Here's how the part is built. I have some questions about the finished solid (model axes, mm). Coordinates: 2 decimals unless noted, no trailing zeros. Use one line per item in the form item = value. Start each with the question number.
(1) Thinking about a two-plate mould opening in Z: for faces 1 (the cylindrical face through (40.926, 1.479, -84.608)), 2 (the flat face through (12, 3, -54)), 3 (the cylindrical face through (13.16, 1.48, 31.19)), 4 (the cylindrical face through (-39.44, 1.52, 36.02)), which applies, +Z half, -Z half, draft (parallel to the pull), parting line (faces both ways), or undercut?
(2) Imagine slicing it at A-A, the plane y = 0.8. State how many separate pieces and enclosed holes the cut face has, and give its area (3 significant figures).
(3) Please list where these lines run through material, in increasing order: L1, parallel to Z at x = 3, y = 1.4; L2, parallel to Z at x = 14, y = 2.3; L3, parallel to Z at x = 62, y = 0.4.
(4) Will these pins go through, and if not, where does the flat tip stop? P1, Ø4, axis at x = 12.63, z = -10.48, coming from the +Y side; P2, Ø2, axis at x = 32.63, z = 29.52, coming from the -Y side.
```python
from build123d import *

# Parameters (mm, degrees)
SKETCH1_W           = 107
SKETCH1_H           = 179.75
SKETCH1_R           = 1.75
BOSS_EXTRUDE1_DEPTH = 3
FILLET1_R           = 5


with BuildPart() as part:
    # Sketch1 → Boss-Extrude1 (new body)
    with BuildSketch(Plane(origin=(0, 0, 0), x_dir=(1, 0, 0), z_dir=(0, 1, 0))):
        with Locations((12.634153991, 52.353571429)):
            Rectangle(SKETCH1_W, SKETCH1_H)
        with Locations(Location((-32.865846009, -22.771428571, 0), (0, 0, 270))):
            Circle(SKETCH1_R, mode=Mode.SUBTRACT)
        with Locations(Location((-32.865846009, 59.728571429, 0), (0, 0, 270))):
            Circle(SKETCH1_R, mode=Mode.SUBTRACT)
        with Locations(Location((-32.865846009, -29.521428571, 0), (0, 0, 270))):
            Circle(SKETCH1_R, mode=Mode.SUBTRACT)
        with Locations(Location((-32.865846009, -16.021428571, 0), (0, 0, 270))):
            Circle(SKETCH1_R, mode=Mode.SUBTRACT)
        with Locations(Location((-32.865846009, 22.978571429, 0), (0, 0, 270))):
            Circle(SKETCH1_R, mode=Mode.SUBTRACT)
        with Locations(Location((-32.865846009, 30.478571429, 0), (0, 0, 270))):
            Circle(SKETCH1_R, mode=Mode.SUBTRACT)
        with Locations(Location((-32.865846009, 71.728571429, 0), (0, 0, 270))):
            Circle(SKETCH1_R, mode=Mode.SUBTRACT)
        with Locations(Location((-32.865846009, 84.228571429, 0), (0, 0, 270))):
            Circle(SKETCH1_R, mode=Mode.SUBTRACT)
        with Locations(Location((-32.865846009, 104.728571429, 0), (0, 0, 270))):
            Circle(SKETCH1_R, mode=Mode.SUBTRACT)
        with Locations(Location((12.634153991, 84.228571429, 0), (0, 0, 270))):
            Circle(SKETCH1_R, mode=Mode.SUBTRACT)
        with Locations(Location((2.634153991, 84.228571429, 0), (0, 0, 270))):
            Circle(SKETCH1_R, mode=Mode.SUBTRACT)
        with Locations(Location((-7.365846009, 84.228571429, 0), (0, 0, 270))):
            Circle(SKETCH1_R, mode=Mode.SUBTRACT)
        with Locations(Location((-17.365846009, 84.228571429, 0), (0, 0, 270))):
            Circle(SKETCH1_R, mode=Mode.SUBTRACT)
        with Locations(Location((-25.115846009, -29.521428571, 0), (0, 0, 270))):
            Circle(SKETCH1_R, mode=Mode.SUBTRACT)
        with Locations(Location((-17.365846009, -29.521428571, 0), (0, 0, 270))):
            Circle(SKETCH1_R, mode=Mode.SUBTRACT)
        with Locations(Location((-7.365846009, -29.521428571, 0), (0, 0, 270))):
            Circle(SKETCH1_R, mode=Mode.SUBTRACT)
        with Locations(Location((2.634153991, -29.521428571, 0), (0, 0, 270))):
            Circle(SKETCH1_R, mode=Mode.SUBTRACT)
        with Locations(Location((12.634153991, -29.521428571, 0), (0, 0, 270))):
            Circle(SKETCH1_R, mode=Mode.SUBTRACT)
        with Locations(Location((-17.365846009, 10.478571429, 0), (0, 0, 270))):
            Circle(SKETCH1_R, mode=Mode.SUBTRACT)
        with Locations(Location((-7.365846009, 10.478571429, 0), (0, 0, 270))):
            Circle(SKETCH1_R, mode=Mode.SUBTRACT)
        with Locations(Location((2.634153991, 10.478571429, 0), (0, 0, 270))):
            Circle(SKETCH1_R, mode=Mode.SUBTRACT)
        with Locations(Location((12.634153991, 10.478571429, 0), (0, 0, 270))):
            Circle(SKETCH1_R, mode=Mode.SUBTRACT)
        with Locations(Location((2.634153991, 133.228571429, 0), (0, 0, 270))):
            Circle(SKETCH1_R, mode=Mode.SUBTRACT)
        with Locations(Location((-7.365846009, 133.228571429, 0), (0, 0, 270))):
            Circle(SKETCH1_R, mode=Mode.SUBTRACT)
        with Locations(Location((12.634153991, 133.228571429, 0), (0, 0, 270))):
            Circle(SKETCH1_R, mode=Mode.SUBTRACT)
        with Locations(Location((-32.865846009, 133.228571429, 0), (0, 0, 270))):
            Circle(SKETCH1_R, mode=Mode.SUBTRACT)
        with Locations(Location((-17.365846009, 133.228571429, 0), (0, 0, 270))):
            Circle(SKETCH1_R, mode=Mode.SUBTRACT)
        with Locations(Location((42.634153991, 133.228571429, 0), (0, 0, 270))):
            Circle(SKETCH1_R, mode=Mode.SUBTRACT)
        with Locations(Location((58.134153991, 133.228571429, 0), (0, 0, 270))):
            Circle(SKETCH1_R, mode=Mode.SUBTRACT)
        with Locations(Location((32.634153991, 133.228571429, 0), (0, 0, 270))):
            Circle(SKETCH1_R, mode=Mode.SUBTRACT)
        with Locations(Location((22.634153991, 133.228571429, 0), (0, 0, 270))):
            Circle(SKETCH1_R, mode=Mode.SUBTRACT)
        with Locations(Location((22.634153991, 10.478571429, 0), (0, 0, 270))):
            Circle(SKETCH1_R, mode=Mode.SUBTRACT)
        with Locations(Location((32.634153991, 10.478571429, 0), (0, 0, 270))):
            Circle(SKETCH1_R, mode=Mode.SUBTRACT)
        with Locations(Location((42.634153991, 10.478571429, 0), (0, 0, 270))):
            Circle(SKETCH1_R, mode=Mode.SUBTRACT)
        with Locations(Location((22.634153991, -29.521428571, 0), (0, 0, 270))):
            Circle(SKETCH1_R, mode=Mode.SUBTRACT)
        with Locations(Location((32.634153991, -29.521428571, 0), (0, 0, 270))):
            Circle(SKETCH1_R, mode=Mode.SUBTRACT)
        with Locations(Location((42.634153991, -29.521428571, 0), (0, 0, 270))):
            Circle(SKETCH1_R, mode=Mode.SUBTRACT)
        with Locations(Location((50.384153991, -29.521428571, 0), (0, 0, 270))):
            Circle(SKETCH1_R, mode=Mode.SUBTRACT)
        with Locations(Location((42.634153991, 84.228571429, 0), (0, 0, 270))):
            Circle(SKETCH1_R, mode=Mode.SUBTRACT)
        with Locations(Location((32.634153991, 84.228571429, 0), (0, 0, 270))):
            Circle(SKETCH1_R, mode=Mode.SUBTRACT)
        with Locations(Location((22.634153991, 84.228571429, 0), (0, 0, 270))):
            Circle(SKETCH1_R, mode=Mode.SUBTRACT)
        with Locations(Location((58.134153991, 104.728571429, 0), (0, 0, 270))):
            Circle(SKETCH1_R, mode=Mode.SUBTRACT)
        with Locations(Location((58.134153991, 84.228571429, 0), (0, 0, 270))):
            Circle(SKETCH1_R, mode=Mode.SUBTRACT)
        with Locations(Location((58.134153991, 71.728571429, 0), (0, 0, 270))):
            Circle(SKETCH1_R, mode=Mode.SUBTRACT)
        with Locations(Location((58.134153991, 30.478571429, 0), (0, 0, 270))):
            Circle(SKETCH1_R, mode=Mode.SUBTRACT)
        with Locations(Location((58.134153991, 22.978571429, 0), (0, 0, 270))):
            Circle(SKETCH1_R, mode=Mode.SUBTRACT)
        with Locations(Location((58.134153991, -16.021428571, 0), (0, 0, 270))):
            Circle(SKETCH1_R, mode=Mode.SUBTRACT)
        with Locations(Location((58.134153991, -29.521428571, 0), (0, 0, 270))):
            Circle(SKETCH1_R, mode=Mode.SUBTRACT)
        with Locations(Location((58.134153991, 59.728571429, 0), (0, 0, 270))):
            Circle(SKETCH1_R, mode=Mode.SUBTRACT)
        with Locations(Location((58.134153991, -22.771428571, 0), (0, 0, 270))):
            Circle(SKETCH1_R, mode=Mode.SUBTRACT)
    extrude(amount=BOSS_EXTRUDE1_DEPTH)

    # Fillet1
    fillet1_edges = [part.edges().sort_by_distance(p)[0] for p in [
        (66.134153991, 1.5, 37.521428571),
        (-40.865846009, 1.5, 37.521428571),
    ]]
    fillet(fillet1_edges, radius=FILLET1_R)


solid = part.part
```
Answer:
q1.face_1 = undercut
q1.face_2 = draft
q1.face_3 = undercut
q1.face_4 = +Z half
q2.separate_pieces = 1
q2.enclosed_holes = 50
q2.area = 18,700 mm²
q3.L1 = -142.23 to -134.94, -131.52 to -85.94, -82.52 to -12.19, -8.77 to 27.81, 31.23 to 37.52
q3.L2 = -142.23 to -134.32, -132.13 to -85.32, -83.13 to -11.57, -9.38 to 28.43, 30.62 to 37.52
q3.L3 = -142.23 to 37.45
q4.P1 = 3
q4.P2 = through
